Here's how the part is built. I have some questions about the finished solid (model axes, mm). Coordinates: 2 decimals unless noted, no trailing zeros. Write each loop counter-clockwise with the first axis right and the second up, starting at its lowest first coordinate (ties: lowest second). Pieces come first, ordered by that corner, then holes. Notation, with made-up numbers: M 84,15.25 L 103,15.25 A18 cw 103,26.25 Z; hole C -26,15.5 d6. An arc over 180 degrees is marked long. Use a Markdown table: item, result.
```python
from build123d import *

# Parameters (mm, degrees)
SKETCH_1_R      = 2.05
SKETCH_1_R_2    = 4
SKETCH_1_R_3    = 2.332988974
SKETCH_1_R_4    = 1.601067765
SKETCH_1_W      = 8.8
SKETCH_1_H      = 2.8
SKETCH_1_W_2    = 2.5
SKETCH_1_H_2    = 8.5
SKETCH_1_W_3    = 8.5
SKETCH_1_H_3    = 2.5
SKETCH_1_W_4    = 241.301375666
SKETCH_1_H_4    = 241.301375666
SKETCH_1_W_5    = 2.3
SKETCH_1_H_5    = 4.3
EXTRUDE_1_DEPTH = 2


with BuildPart() as part:
    # 草图1 → 凸台-拉伸1 (new body)
    with BuildSketch(Plane.XY):
        Polygon((-150.650687833, -150.650687833), (-150.650687833, 150.650687833), (150.650687833, 150.650687833), (200.650687833, 150.650687833), (200.650687833, -278.650687833), (150.650687833, -278.650687833), (-150.650687833, -278.650687833), align=None)
        with Locations((0.724285714, -142.895)):
            Circle(SKETCH_1_R, mode=Mode.SUBTRACT)
        with Locations((66.724285714, -142.895)):
            Circle(SKETCH_1_R, mode=Mode.SUBTRACT)
        with Locations((-65.275714286, -142.895)):
            Circle(SKETCH_1_R, mode=Mode.SUBTRACT)
        with Locations((-143.125714286, 66.955)):
            Circle(SKETCH_1_R, mode=Mode.SUBTRACT)
        with Locations((-143.125714286, 0.955)):
            Circle(SKETCH_1_R, mode=Mode.SUBTRACT)
        with Locations((-143.125714286, -65.045)):
            Circle(SKETCH_1_R, mode=Mode.SUBTRACT)
        with Locations((66.874285714, 144.955)):
            Circle(SKETCH_1_R, mode=Mode.SUBTRACT)
        with Locations((0.874285714, 144.955)):
            Circle(SKETCH_1_R, mode=Mode.SUBTRACT)
        with Locations((-65.125714286, 144.955)):
            Circle(SKETCH_1_R, mode=Mode.SUBTRACT)
        with Locations((144.874285714, -65.045)):
            Circle(SKETCH_1_R, mode=Mode.SUBTRACT)
        with Locations((144.874285714, 0.955)):
            Circle(SKETCH_1_R, mode=Mode.SUBTRACT)
        with Locations((144.874285714, 66.955)):
            Circle(SKETCH_1_R, mode=Mode.SUBTRACT)
        with Locations((-130.650687833, -130.650687833)):
            Circle(SKETCH_1_R_2, mode=Mode.SUBTRACT)
        with Locations((-130.650687833, 130.650687833)):
            Circle(SKETCH_1_R_2, mode=Mode.SUBTRACT)
        with Locations((130.650687833, 130.650687833)):
            Circle(SKETCH_1_R_2, mode=Mode.SUBTRACT)
        with Locations((130.650687833, -130.650687833)):
            Circle(SKETCH_1_R_2, mode=Mode.SUBTRACT)
        with Locations((128.234921063, 21.045946403)):
            Circle(SKETCH_1_R_3, mode=Mode.SUBTRACT)
        with Locations((133.709191973, -41.76906745)):
            Circle(SKETCH_1_R_4, mode=Mode.SUBTRACT)
        with Locations((99.724285714, -142.895)):
            Rectangle(SKETCH_1_W, SKETCH_1_H, mode=Mode.SUBTRACT)
        with Locations((33.724285714, -142.895)):
            Rectangle(SKETCH_1_W, SKETCH_1_H, mode=Mode.SUBTRACT)
        with Locations((-32.275714286, -142.895)):
            Rectangle(SKETCH_1_W, SKETCH_1_H, mode=Mode.SUBTRACT)
        with Locations((-98.275714286, -142.895)):
            Rectangle(SKETCH_1_W, SKETCH_1_H, mode=Mode.SUBTRACT)
        with Locations((-143.125714286, 99.955)):
            Rectangle(SKETCH_1_W_2, SKETCH_1_H_2, mode=Mode.SUBTRACT)
        with Locations((-143.125714286, 33.955)):
            Rectangle(SKETCH_1_W_2, SKETCH_1_H_2, mode=Mode.SUBTRACT)
        with Locations((-143.125714286, -32.045)):
            Rectangle(SKETCH_1_W_2, SKETCH_1_H_2, mode=Mode.SUBTRACT)
        with Locations((-143.125714286, -98.045)):
            Rectangle(SKETCH_1_W_2, SKETCH_1_H_2, mode=Mode.SUBTRACT)
        with Locations((99.874285714, 144.955)):
            Rectangle(SKETCH_1_W_3, SKETCH_1_H_3, mode=Mode.SUBTRACT)
        with Locations((33.874285714, 144.955)):
            Rectangle(SKETCH_1_W_3, SKETCH_1_H_3, mode=Mode.SUBTRACT)
        with Locations((-32.125714286, 144.955)):
            Rectangle(SKETCH_1_W_3, SKETCH_1_H_3, mode=Mode.SUBTRACT)
        with Locations((-98.125714286, 144.955)):
            Rectangle(SKETCH_1_W_3, SKETCH_1_H_3, mode=Mode.SUBTRACT)
        with Locations((144.874285714, -98.045)):
            Rectangle(SKETCH_1_W_2, SKETCH_1_H_2, mode=Mode.SUBTRACT)
        with Locations((144.874285714, -32.045)):
            Rectangle(SKETCH_1_W_2, SKETCH_1_H_2, mode=Mode.SUBTRACT)
        with Locations((144.874285714, 33.955)):
            Rectangle(SKETCH_1_W_2, SKETCH_1_H_2, mode=Mode.SUBTRACT)
        with Locations((144.874285714, 99.955)):
            Rectangle(SKETCH_1_W_2, SKETCH_1_H_2, mode=Mode.SUBTRACT)
        Rectangle(SKETCH_1_W_4, SKETCH_1_H_4, mode=Mode.SUBTRACT)
        with Locations((-146.175714286, -272.895)):
            Rectangle(SKETCH_1_W_5, SKETCH_1_H_5, mode=Mode.SUBTRACT)
        with Locations((-146.175714286, -264.895)):
            Rectangle(SKETCH_1_W_5, SKETCH_1_H_5, mode=Mode.SUBTRACT)
        with Locations((-146.175714286, -164.895)):
            Rectangle(SKETCH_1_W_5, SKETCH_1_H_5, mode=Mode.SUBTRACT)
    extrude(amount=EXTRUDE_1_DEPTH)


solid = part.part
```
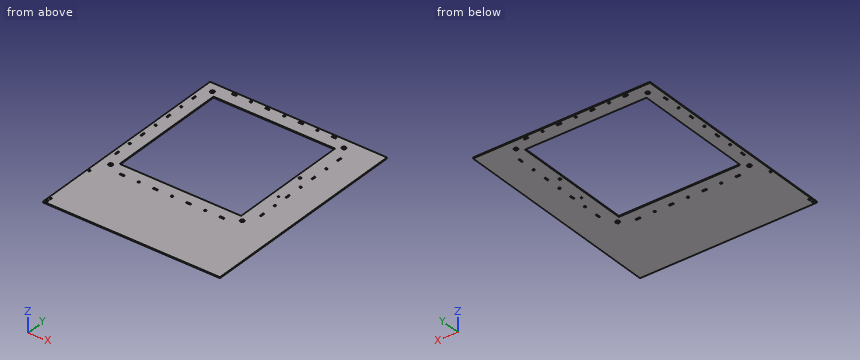
1. Suppose I cut it at C-C on z = 1.1. State how many separate pieces and enclosed holes the cut face has, and give its area (3 significant figures).
Answers follow:
| item | result |
|---|---|
| separate pieces | 1 |
| enclosed holes | 38 |
| area | 91,800 mm2 |
2. Suppose I cut it at B-B on x = 11. Write out the boundary of the cut face in (y, z).
Answers follow:
| item | result |
|---|---|
| outline | M -278.65,0 L -120.65,0 L -120.65,2 L -278.65,2 Z; M 120.65,0 L 150.65,0 L 150.65,2 L 120.65,2 Z |
3. I need wall thicknesses on probe 1 along Y at (x, z) = (36, 1.6) (3 decimals); probe 2 along Y at (x, z) = (-52.5, 0.95); probe 3 along X at (y, z) = (28.5, 1.45). Which ranges of each line are inside material? Lowest first, please.
Answers follow:
| item | result |
|---|---|
| probe 1 | y = -278.651 to -144.295, -141.495 to -120.651, 120.651 to 143.705, 146.205 to 150.651 |
| probe 2 | y = -278.65 to -120.65, 120.65 to 150.65 |
| probe 3 | x = -150.65 to -120.65, 120.65 to 200.65 |
4. Suppose I cut it at A-A on y = 59. Write out the boundary of the cut face in (x, z), and give its area (3 significant figures).
Answers follow:
| item | result |
|---|---|
| outline | M -150.65,0 L -120.65,0 L -120.65,2 L -150.65,2 Z; M 120.65,0 L 200.65,0 L 200.65,2 L 120.65,2 Z |
| area | 220 mm2 |
